from build123d import *

# Parameters (mm, degrees)
F1_DEPTH = 38.1
F3_DEPTH = 3.175
F4_R     = 1.524
F5_R     = 2.54
F5_R_2   = 1.651
F6_DEPTH = 3.175


with BuildPart() as f1:
    # F0 (on Right) → F1 (new body)
    with BuildSketch(Plane.YZ):
        with BuildLine():
            Line((-64.0291666667, 0), (-60.8541666667, 0))
            Line((-60.8541666667, 0), (-60.8541666667, 39.243))
            ThreePointArc((-60.8541666667, 39.243), (-60.4077974012, 40.3206307345), (-59.3301666667, 40.767))
            Line((-59.3301666667, 40.767), (-0.5291666667, 40.767))
            Line((-0.5291666667, 40.767), (-0.5291666667, 43.942))
            Line((-0.5291666667, 43.942), (-59.3301666667, 43.942))
            ThreePointArc((-59.3301666667, 43.942), (-62.6528614315, 42.5656947648), (-64.0291666667, 39.243))
            Line((-64.0291666667, 39.243), (-64.0291666667, 0))
        make_face()
    extrude(amount=F1_DEPTH)

    # F2 (on face) → F3 (cut, through all)
    with BuildSketch(Plane.XZ.offset(64.0291666667)):
        with BuildLine():
            Line((8.89, 31.242), (8.89, 0))
            Line((8.89, 0), (29.21, 0))
            Line((29.21, 0), (29.21, 31.242))
            ThreePointArc((29.21, 31.242), (29.1356051224, 31.4216051224), (28.956, 31.496))
            Line((28.956, 31.496), (9.144, 31.496))
            ThreePointArc((9.144, 31.496), (8.9643948776, 31.4216051224), (8.89, 31.242))
        make_face()
    extrude(amount=-F3_DEPTH, mode=Mode.SUBTRACT)

    # F4
    f4_edges = [f1.edges().sort_by_distance(p)[0] for p in [
        (8.89, -62.441667, 0),
        (0, -62.441667, 0),
        (29.21, -62.441667, 0),
        (38.1, -62.441667, 0),
        (38.1, -0.529167, 42.3545),
        (0, -0.529167, 42.3545),
    ]]
    fillet(f4_edges, radius=F4_R)

    # F5 (on face) → F6 (cut, through all)
    with BuildSketch(Plane.XY.offset(43.942)):
        with Locations((19.05, -8.1491666667)):
            Circle(F5_R)
        with Locations((19.05, -39.8991666667)):
            Circle(F5_R)
        with Locations((31.877, -44.0901666667)):
            Circle(F5_R_2)
        with Locations((6.223, -44.0901666667)):
            Circle(F5_R_2)
    extrude(amount=-F6_DEPTH, mode=Mode.SUBTRACT)


solid = f1.part
Design review of the part built by this model. Coordinates are the model's own, in mm. A direction names the side the tool comes from. Coordinates: 2 decimals unless noted, no trailing zeros. Write each loop counter-clockwise with the first axis right and the second up, starting at its lowest first coordinate (ties: lowest second). Pieces come first, ordered by that corner, then holes. Notation, with made-up numbers: (47, 49) - (54, 49) arc R27 cw to (54, 87) - close; hole circle Ø9 at (-26, 28.5). An arc over 180 degrees is marked (long way). Use one line per item in the form item = value.
Q1. Consider section B-B (y = -6.5). Write out the cut boundary in (x, z).
Taken from the geometry:
outline = (0, 40.77) - (17.12, 40.77) - (17.12, 43.94) - (0, 43.94) - close; (20.98, 40.77) - (38.1, 40.77) - (38.1, 43.94) - (20.98, 43.94) - close
Q2. For probe 1 along Y at (x, z) = (36, 35.5); probe 2 along Z at (x, y) = (10, -57.5); probe 3 along Y at (x, z) = (19.05, 41.95), list the stretches that pass through material, from the lowest coordinate up.
Taken from the geometry:
probe_1 = -64.03 to -60.85
probe_2 = 40.77 to 43.94
probe_3 = -63.17 to -42.44, -37.36 to -10.69, -5.61 to -0.53
Q3. Consider section D-D (y = -25.5). Write out the cut boundary in (x, z), plus the area to 3 significant figures.
Taken from the geometry:
outline = (0, 40.77) - (38.1, 40.77) - (38.1, 43.94) - (0, 43.94) - close
area = 121 mm^2
Q4. Consider section C-C (x = 14.5). Write out the cut boundary in (y, z).
Taken from the geometry:
outline = (-64.03, 31.5) - (-60.85, 31.5) - (-60.85, 39.24) arc R1.52 cw to (-59.33, 40.77) - (-0.53, 40.77) - (-0.53, 43.94) - (-59.33, 43.94) arc R4.7 ccw to (-64.03, 39.24) - close
Q5. Machinability: for faces 4 (the cylindrical face through (8.432, -62.419, 0.435)), 5 (the cylindrical face through (18.5, -42.38, 42.38)), 6 (the flat face through (19, -60.854, 32)), which of the approach directions +Z, -Z, +X, -X, +Y, -Y give a long, thin tool a straight path to every point of the face, cutting with its end or side? Answer none if there is none.
Taken from the geometry:
face_4 = -Z, +Y, -Y
face_5 = +Z, -Z
face_6 = -Z, +X, -X, +Y
Q6. Insertion check: pin 1 Ø3.5 at (x, y) = (24, -62.5) entering from -Z; pin 2 Ø10 at (x, z) = (31.5, 11) entering from +Y; pin 3 Ø11.5 at (x, y) = (21.5, -18.5) entering from -Z. Each pin has a flat end and moves straight along its axis. Give the tip position at first contact, or say it passes through.
Taken from the geometry:
pin_1 = 31.5
pin_2 = -60.85
pin_3 = 40.77
Q7. Consider section A-A (x = 19.05). Write out the cut boundary in (y, z), plus the area to 3 significant figures.
Taken from the geometry:
outline = (-64.03, 31.5) - (-60.85, 31.5) - (-60.85, 39.24) arc R1.52 cw to (-59.33, 40.77) - (-42.44, 40.77) - (-42.44, 43.94) - (-59.33, 43.94) arc R4.7 ccw to (-64.03, 39.24) - close; (-37.36, 40.77) - (-10.69, 40.77) - (-10.69, 43.94) - (-37.36, 43.94) - close; (-5.61, 40.77) - (-0.53, 40.77) - (-0.53, 43.94) - (-5.61, 43.94) - close
area = 195 mm^2
Q8. The part is to be moulded in two halves that separate along X. For faces 1 (the cylindrical face through (31.519, -45.702, 42.377)), 2 (the cylindrical face through (18.78, -60.42, 40.31)), 3 (the flat face through (0, -42, 42)), say which applies: +X half, -X half, draft (parallel to the pull), parting line (faces both ways), or undercut.
Taken from the geometry:
face_1 = undercut
face_2 = draft
face_3 = -X half
